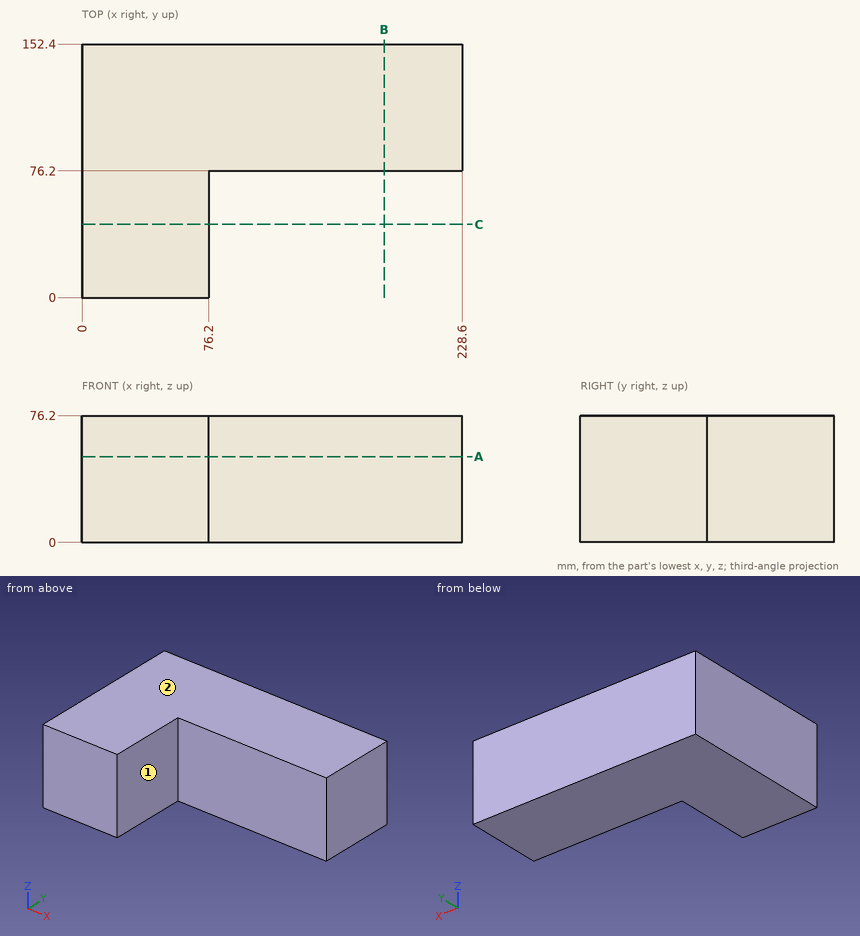
Study the drawing (mm; zero at the part's minimum x, y, z) and answer. A direction names the side the tool comes from. Round coordinates to 2 decimals unless told otherwise and drop trailing zeros. Write each loop counter-clockwise with the first axis right and the second up, starting at its lowest first coordinate (ties: lowest second). Pieces come first, ordered by that corner, then holes.
Q1. Straight lines are drawn through the part: line 1 (X direction, y = 42, z = 46.5); line 2 (Y direction, x = 88, z = 58.5). For each, find the intervals that lie inside material, in ascending order.
Values:
line 1: x = 0 to 76.2
line 2: y = 76.2 to 152.4
Q2. Find section B-B on x = 181.5. Determine the outline of the cut face in (y, z).
Values:
outline: (76.2, 0) - (152.4, 0) - (152.4, 76.2) - (76.2, 76.2) - close
Q3. A flat-ended cylindrical pin translates along its axis: P1, Ø6, axis at x = 200.5, z = 53.5, coming from the -Y side. Find the tip coordinate at first contact, or state that the pin passes through.
Values:
P1: stops at y = 76.2
Q4. Find section A-A on z = 51.5. Determine the outline of the cut face in (x, y).
Values:
outline: (0, 0) - (76.2, 0) - (76.2, 76.2) - (228.6, 76.2) - (228.6, 152.4) - (0, 152.4) - close
Q5. A tool of negligible diameter and unlimited length cuts with its end or side. For the marked faces 1 and 2, from which of +Z, -Z, +X, -X, +Y, -Y can it reach the whole face along a straight path? Write none if from no direction.
Values:
face 1: +Z, -Z, +X, -Y
face 2: +Z, +X, -X, +Y, -Y
Q6. Find section C-C on y = 44. Determine the outline of the cut face in (x, z), and give its area (3 significant figures).
Values:
outline: (0, 0) - (76.2, 0) - (76.2, 76.2) - (0, 76.2) - close
area: 5,810 mm2
